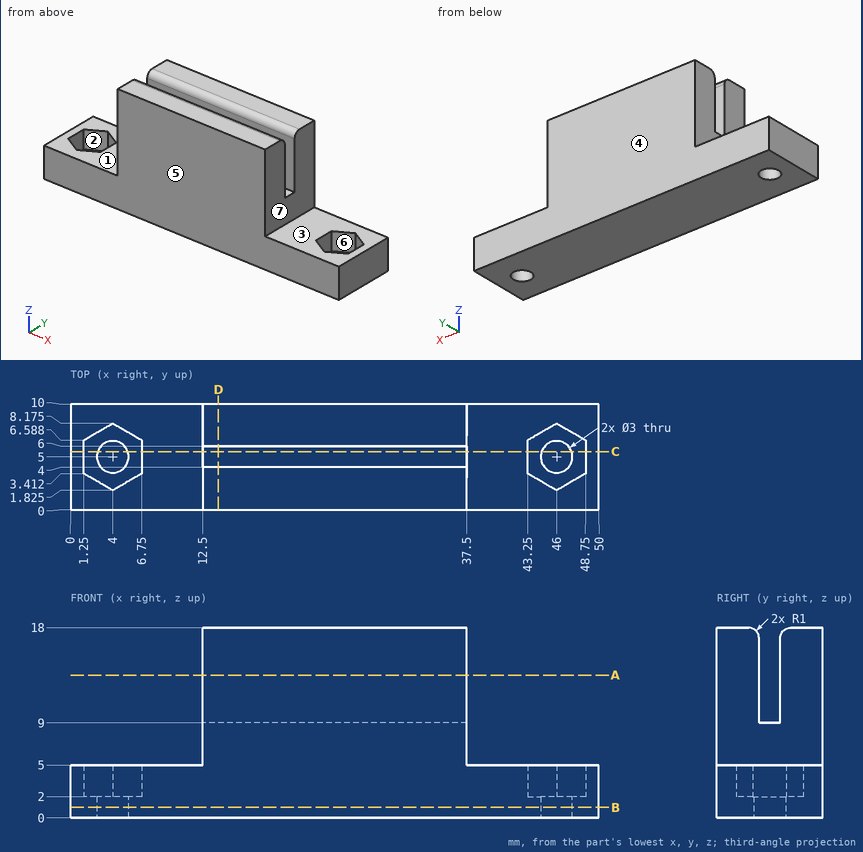
Print and shaded views of the part. All mm, measured from the part's lowest x, y and z. A direction names the side the tool comes from. Round coordinates to 2 decimals unless told otherwise and drop trailing zeros. Write each loop counter-clockwise with the first axis right and the second up, starting at its lowest first coordinate (ties: lowest second). Pieces come first, ordered by that corner, then holes.
(1) Slice it at D-D, the plane x = 14. Write the cut outline in (y, z).
(2) Drop flat-ended pins along their axis: P1, Ø3, axis at y = 3.5, z = 14.5, coming from the +X side; P2, Ø1.6, axis at x = 2.5, y = 3.5, coming from the +Z side; P3, Ø3, axis at x = 46.5, y = 6, coming from the +Z side. Give the stop position or say it passes through.
(3) Mould opens along Y. For the marked faces 4, 5, 6 and 7 say: pulls with the +Y half, pulls with the -Y half, needs draft (parallel to the pull), parting line crosses it, or undercut.
(4) 3-axis set-ups, long thin cutter, end or side, ignore diameter. For the marked faces 1, 2 and 3: which of +Z, -Z, +X, -X, +Y, -Y reach the whole face in a straight line?
(5) Slice it at A-A, the plane z = 13.5. Write the cut outline in (x, y).
(6) Slice it at B-B, the plane z = 1. Write the cut outline in (x, y).
(7) Probe line 1 along X through (y, z) = (4, 2.25); line 2 along Y through (x, z) = (4, 1.55); line 3 along X through (y, z) = (6.25, 9.5). List the from-to ranges inside material, lowest first.
(8) Slice it at C-C, the plane y = 5.5. Count the separate pieces of the cut face and the enclosed holes in it, and give its area (3 significant figures).
From the geometry:
1. outline: (0, 0) - (10, 0) - (10, 18) - (7, 18) arc R1 ccw to (6, 17) - (6, 9) - (4, 9) - (4, 17) arc R1 ccw to (3, 18) - (0, 18) - close
2. P1: stops at x = 37.5
2. P2: stops at z = 5
2. P3: stops at z = 2
3. face 4: pulls with the +Y half
3. face 5: pulls with the -Y half
3. face 6: undercut
3. face 7: needs draft
4. face 1: +Z, -X, +Y, -Y
4. face 2: +Z
4. face 3: +Z, +X, +Y, -Y
5. outline: (12.5, 0) - (37.5, 0) - (37.5, 4) - (12.5, 4) - close; (12.5, 6) - (37.5, 6) - (37.5, 10) - (12.5, 10) - close
6. outline: (0, 0) - (50, 0) - (50, 10) - (0, 10) - close; hole circle Ø3 at (4, 5); hole circle Ø3 at (46, 5)
7. line 1: x = 0 to 1.25, 6.75 to 43.25, 48.75 to 50
7. line 2: y = 0 to 3.5, 6.5 to 10
7. line 3: x = 12.5 to 37.5
8. separate pieces: 3
8. enclosed holes: 0
8. area: 306 mm2
